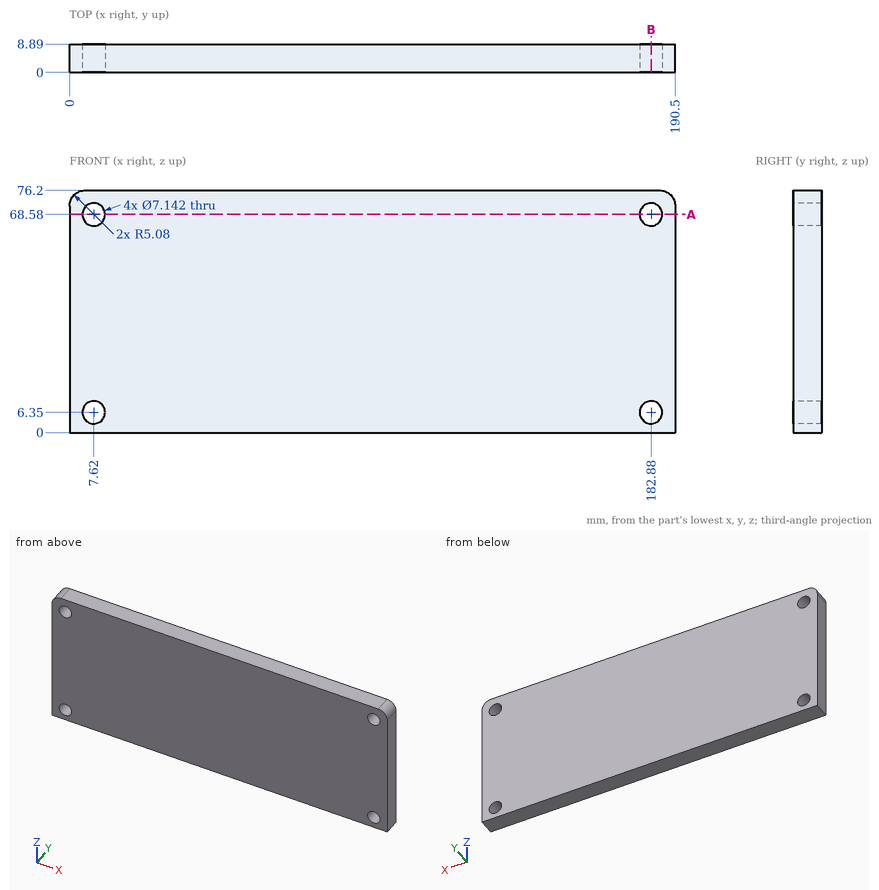
Here's the drawing with two shaded views (mm, measured from the low corner). I have some questions. Coordinates: 2 decimals unless noted, no trailing zeros. Loops run counter-clockwise (first coordinate to the right, second up) from the corner with the lowest first, then second, coordinate; pieces in that order, holes last. Notation, with made-up numbers: M 32,81.25 L 81,81.25 A14 cw 81,108.25 Z; hole C 59,-14 d2. An arc over 180 degrees is marked long. Put each result on its own line as item: value. Start each with the question number.
(1) I need wall thicknesses on probe 1 along Z at (x, y) = (7.62, 2.5); probe 2 along X at (y, z) = (2.5, 6.5); probe 3 along X at (y, z) = (2.5, 67). Which ranges of each line are inside material? Lowest first, please.
(2) Imagine slicing it at B-B on x = 182.88. List the corners of the cut face in (y, z) for me.
(3) Imagine slicing it at A-A on z = 68.58. List the corners of the cut face in (x, y) for me, and give its area (3 significant figures).
Worked answers:
1. probe 1: z = 0 to 2.78, 9.92 to 65.01, 72.15 to 76.2
1. probe 2: x = 0 to 4.05, 11.19 to 179.31, 186.45 to 190.5
1. probe 3: x = 0 to 4.42, 10.82 to 179.68, 186.08 to 190.5
2. outline: M 0,0 L 8.89,0 L 8.89,2.78 L 0,2.78 Z; M 0,9.92 L 8.89,9.92 L 8.89,65.01 L 0,65.01 Z; M 0,72.15 L 8.89,72.15 L 8.89,76.2 L 0,76.2 Z
3. outline: M 0,0 L 4.05,0 L 4.05,8.89 L 0,8.89 Z; M 11.19,0 L 179.31,0 L 179.31,8.89 L 11.19,8.89 Z; M 186.45,0 L 190.5,0 L 190.5,8.89 L 186.45,8.89 Z
3. area: 1,570 mm2
